Work out the finished part from the listing and answer in its coordinate system (mm). Face numbers are marked on the shaded views. A direction names the side the tool comes from. Coordinates: 2 decimals unless noted, no trailing zeros. Write each loop counter-clockwise with the first axis right and the second up, starting at its lowest first coordinate (ties: lowest second). Pieces come first, ordered by that corner, then holes. Notation, with made-up numbers: (35.5, -8) - (78.5, -8) arc R14 ccw to (78.5, 11) - close; hole circle Ø8 at (0, 39.25). An arc over 180 degrees is marked (long way). One line per item, written item: value.
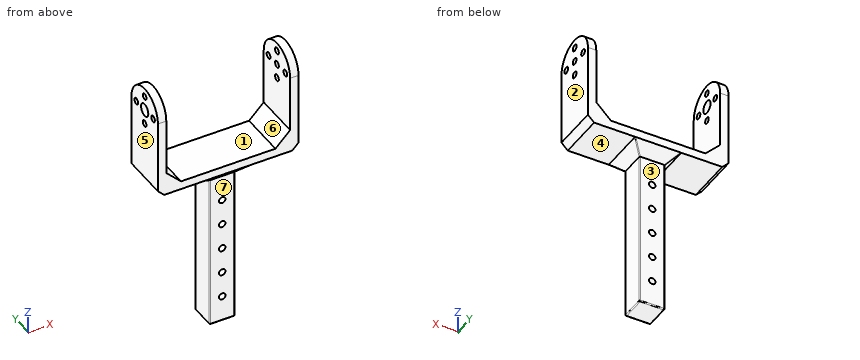
```python
from build123d import *

# Parameters (mm, degrees)
BOSS_EXTRUDE1_DEPTH      = 22
SKETCH3_R                = 1.55
CUT_EXTRUDE1_DEPTH       = 30
CUT_EXTRUDE5_DEPTH       = 9
SKETCH11_R               = 1.55
CUT_EXTRUDE10_DEPTH      = 13
CUT_EXTRUDE11_START      = -10
CUT_EXTRUDE11_DEPTH      = 10
SKETCH13_R               = 3
SKETCH13_R_2             = 1.5
CUT_EXTRUDE12_DEPTH      = 4
SKETCH14_W               = 54
SKETCH14_H               = 9.3
SKETCH14_W_2             = 7.05
SKETCH14_H_2             = 4
BOSS_EXTRUDE4_DEPTH      = 4
SKETCH17_W               = 7.05
SKETCH17_H               = 4
BOSS_EXTRUDE5_DEPTH      = 23.05
BOSS_EXTRUDE6_DEPTH      = 27.3
BOSS_EXTRUDE6_DEPTH_BACK = 4
SKETCH18_W               = 54
SKETCH18_H               = 2.95
SKETCH19_W               = 54
SKETCH19_H               = 2.8
BOSS_EXTRUDE7_DEPTH      = 21
FILLET2_SIZE             = 6.5
FILLET3_SIZE             = 0.5
SKETCH20_R               = 3.970030919
BOSS_EXTRUDE8_DEPTH      = 6
FILLET4_R                = 1
CUT_EXTRUDE13_START      = -37.3
CUT_EXTRUDE13_DEPTH      = 37.3
SKETCH22_W               = 56.118071471
SKETCH22_H               = 11.813110758
CUT_EXTRUDE14_DEPTH      = 56
SKETCH23_W               = 67
SKETCH23_H               = 4
BOSS_EXTRUDE9_DEPTH      = 4
SKETCH24_W               = 67
SKETCH24_H               = 4
BOSS_EXTRUDE10_DEPTH     = 4
SKETCH25_W               = 12
SKETCH25_H               = 12
BOSS_EXTRUDE11_DEPTH     = 80
FILLET6_SIZE             = 7
SKETCH27_W               = 67
SKETCH27_H               = 4
CUT_EXTRUDE16_DEPTH      = 80
FILLET7_SIZE             = 5
SKETCH29_R               = 1.55
CUT_EXTRUDE17_DEPTH      = 12
FILLET8_R                = 0.5
FILLET9_R                = 0.5
FILLET10_SIZE            = 3


# Read off the part's stored shape, not the designer's step: Cut-Extrude13
with BuildPart() as part:
    # Sketch1 → Boss-Extrude1 (new body)
    with BuildSketch(Plane(origin=(0, 0, 0), x_dir=(1, 0, 0), z_dir=(0, 1, 0))):
        Polygon((0, 0), (0, 50), (67, 50), (67, 0), (63, 0), (63, 46), (4, 46), (4, 0), align=None)
    extrude(amount=BOSS_EXTRUDE1_DEPTH)

    # Sketch3 → Cut-Extrude1 (cut)
    with BuildSketch(Plane(origin=(67, 0, 0), x_dir=(0, 0, -1), z_dir=(1, 0, 0))):
        with Locations((12.05, 11)):
            Circle(SKETCH3_R)
    extrude(amount=-CUT_EXTRUDE1_DEPTH, mode=Mode.SUBTRACT)

    # Sketch5 → Cut-Extrude5 (cut)
    with BuildSketch(Plane(origin=(67, 0, 0), x_dir=(0, 0, -1), z_dir=(1, 0, 0))):
        with BuildLine():
            Line((12.05, 22), (0, 22))
            Line((0, 22), (0, 0))
            Line((0, 0), (12.05, 0))
            ThreePointArc((12.05, 0), (1.05, 11), (12.05, 22))
        make_face()
    extrude(amount=-CUT_EXTRUDE5_DEPTH, mode=Mode.SUBTRACT)

    # Sketch11 → Cut-Extrude10 (cut)
    with BuildSketch(Plane(origin=(67, 0, 0), x_dir=(0, 0, -1), z_dir=(1, 0, 0))):
        with Locations((19.05, 11)):
            Circle(SKETCH11_R)
        with Locations((12.05, 18)):
            Circle(SKETCH11_R)
        with Locations((12.05, 4)):
            Circle(SKETCH11_R)
        with Locations((5.05, 11)):
            Circle(SKETCH11_R)
    extrude(amount=-CUT_EXTRUDE10_DEPTH, mode=Mode.SUBTRACT)

    # Sketch12 → Cut-Extrude11 (cut)
    with BuildSketch(Plane.ZY.offset(CUT_EXTRUDE11_START)):
        with BuildLine():
            Line((-12.05, 22), (0, 22))
            Line((0, 22), (0, 0))
            Line((0, 0), (-12.05, 0))
            ThreePointArc((-12.05, 0), (-1.05, 11), (-12.05, 22))
        make_face()
    extrude(amount=CUT_EXTRUDE11_DEPTH, mode=Mode.SUBTRACT)

    # Sketch13 → Cut-Extrude12 (cut)
    with BuildSketch(Plane.ZY):
        with Locations((-12.05, 11)):
            Circle(SKETCH13_R)
        with Locations((-19.05, 11)):
            Circle(SKETCH13_R_2)
        with Locations((-12.05, 4)):
            Circle(SKETCH13_R_2)
        with Locations((-5.05, 11)):
            Circle(SKETCH13_R_2)
        with Locations((-12.05, 18)):
            Circle(SKETCH13_R_2)
    extrude(amount=-CUT_EXTRUDE12_DEPTH, mode=Mode.SUBTRACT)

    # Sketch14 → Boss-Extrude4 (add)
    with BuildSketch(Plane(origin=(0, 0, -50), x_dir=(-1, 0, 0), z_dir=(0, 0, -1))):
        with Locations((-33.5, -4.65)):
            Rectangle(SKETCH14_W, SKETCH14_H)
        with Locations((-56.975, 20)):
            Rectangle(SKETCH14_W_2, SKETCH14_H_2)
        with Locations((-10.025, 20)):
            Rectangle(SKETCH14_W_2, SKETCH14_H_2)
    extrude(amount=-BOSS_EXTRUDE4_DEPTH)

    # Sketch17 → Boss-Extrude5 (add)
    with BuildSketch(Plane(origin=(0, 0, -50), x_dir=(-1, 0, 0), z_dir=(0, 0, -1))):
        with Locations((-56.975, 20)):
            Rectangle(SKETCH17_W, SKETCH17_H)
        with Locations((-10.025, 20)):
            Rectangle(SKETCH17_W, SKETCH17_H)
    extrude(amount=BOSS_EXTRUDE5_DEPTH)

    # Sketch18 → Boss-Extrude6 (add, two sides: drawn at the far end of the back side and taken through both)
    with BuildSketch(Plane.XZ.offset(-18).offset(-BOSS_EXTRUDE6_DEPTH_BACK)):
        with Locations((33.5, -71.575)):
            Rectangle(SKETCH18_W, SKETCH18_H)
    extrude(amount=BOSS_EXTRUDE6_DEPTH + BOSS_EXTRUDE6_DEPTH_BACK)

    # Sketch19 → Boss-Extrude7 (add)
    with BuildSketch(Plane(origin=(0, 0, -50), x_dir=(-1, 0, 0), z_dir=(0, 0, -1))):
        with Locations((-33.5, -7.9)):
            Rectangle(SKETCH19_W, SKETCH19_H)
    extrude(amount=BOSS_EXTRUDE7_DEPTH)

    # Fillet2
    fillet2_edges = [part.edges().sort_by_distance(p)[0] for p in [
        (60.5, 20, -50),
        (6.5, 20, -50),
    ]]
    chamfer(fillet2_edges, length=FILLET2_SIZE - 0.0001)  # a hair under: the kernel refuses the full size

    # Fillet3
    fillet3_edges = [part.edges().sort_by_distance(p)[0] for p in [
        (60.5, 6.35, -73.05),
        (6.5, 6.35, -73.05),
    ]]
    chamfer(fillet3_edges, length=FILLET3_SIZE)

    # Sketch20 → Boss-Extrude8 (add)
    with BuildSketch(Plane.XZ.offset(9.3)):
        with Locations(Location((23.4, -59.65, 0), (0, 0, 270))):
            Circle(SKETCH20_R)
    extrude(amount=BOSS_EXTRUDE8_DEPTH)

    # Fillet4
    fillet4_edges = [part.edges().sort_by_distance(p)[0] for p in [
        (23.4, -15.3, -55.679969081),
    ]]
    fillet(fillet4_edges, radius=FILLET4_R)

    # Cut-Extrude13 outline → Cut-Extrude13 (cut)
    with BuildSketch(Plane(origin=(0, 22, 0), x_dir=(1, 0, 0), z_dir=(0, 1, 0)).offset(CUT_EXTRUDE13_START)):
        Polygon((67, 50), (60.5, 56.5), (60.5, 72.55), (60, 73.05), (7, 73.05), (6.5, 72.55), (6.5, 56.5), (0, 50), align=None)
    extrude(amount=CUT_EXTRUDE13_DEPTH, mode=Mode.SUBTRACT)

    # Sketch22 → Cut-Extrude14 (cut)
    with BuildSketch(Plane(origin=(0, 0, -50), x_dir=(-1, 0, 0), z_dir=(0, 0, -1))):
        with Locations((-32.440964265, -5.906555379)):
            Rectangle(SKETCH22_W, SKETCH22_H)
    extrude(amount=-CUT_EXTRUDE14_DEPTH, mode=Mode.SUBTRACT)

    # Sketch23 → Boss-Extrude9 (add)
    with BuildSketch(Plane(origin=(0, 22, 0), x_dir=(1, 0, 0), z_dir=(0, 1, 0))):
        with Locations((33.5, 48)):
            Rectangle(SKETCH23_W, SKETCH23_H)
    extrude(amount=BOSS_EXTRUDE9_DEPTH)

    # Sketch24 → Boss-Extrude10 (add)
    with BuildSketch(Plane.XZ):
        with Locations((33.5, -48)):
            Rectangle(SKETCH24_W, SKETCH24_H)
    extrude(amount=BOSS_EXTRUDE10_DEPTH)

    # Sketch25 → Boss-Extrude11 (add)
    with BuildSketch(Plane(origin=(0, 0, -50), x_dir=(-1, 0, 0), z_dir=(0, 0, -1))):
        with Locations((-33.5, 11)):
            Rectangle(SKETCH25_W, SKETCH25_H)
    extrude(amount=BOSS_EXTRUDE11_DEPTH)

    # Fillet6
    fillet6_edges = [part.edges().sort_by_distance(p)[0] for p in [
        (63, 11, -46),
        (4, 11, -46),
    ]]
    chamfer(fillet6_edges, length=FILLET6_SIZE)

    # Sketch27 → Cut-Extrude16 (cut)
    with BuildSketch(Plane.XY.offset(-46)):
        with Locations((33.5, 24)):
            Rectangle(SKETCH27_W, SKETCH27_H)
        with Locations((33.5, -2)):
            Rectangle(SKETCH27_W, SKETCH27_H)
    extrude(amount=-CUT_EXTRUDE16_DEPTH, mode=Mode.SUBTRACT)

    # Fillet7
    fillet7_edges = [part.edges().sort_by_distance(p)[0] for p in [
        (39.5, 11, -50),
        (33.5, 5, -50),
        (27.5, 11, -50),
        (33.5, 17, -50),
    ]]
    chamfer(fillet7_edges, length=FILLET7_SIZE - 0.0001)  # a hair under: the kernel refuses the full size

    # Sketch29 → Cut-Extrude17 (cut)
    with BuildSketch(Plane.XZ.offset(-5)):
        with Locations(Location((33.5, -67.5, 0), (0, 0, 270))):
            Circle(SKETCH29_R)
        with Locations(Location((33.5, -80, 0), (0, 0, 270))):
            Circle(SKETCH29_R)
        with Locations(Location((33.5, -92.5, 0), (0, 0, 270))):
            Circle(SKETCH29_R)
        with Locations(Location((33.5, -105, 0), (0, 0, 270))):
            Circle(SKETCH29_R)
        with Locations(Location((33.5, -117.5, 0), (0, 0, 270))):
            Circle(SKETCH29_R)
    extrude(amount=-CUT_EXTRUDE17_DEPTH, mode=Mode.SUBTRACT)

    # Fillet8
    fillet8_edges = [part.edges().sort_by_distance(p)[0] for p in [
        (39.5, 17, -92.49995),
        (39.5, 5, -92.49995),
        (27.5, 5, -92.49995),
        (27.5, 17, -92.49995),
        (39.5, 11, -130),
        (33.5, 5, -130),
        (27.5, 11, -130),
        (33.5, 17, -130),
    ]]
    fillet(fillet8_edges, radius=FILLET8_R)

    # Fillet9
    fillet9_edges = [part.edges().sort_by_distance(p)[0] for p in [
        (41.926726695, 19.426726695, -52.573173305),
        (41.926726695, 2.573273305, -52.573173305),
        (25.073273305, 19.426726695, -52.573173305),
        (25.073273305, 2.573273305, -52.573173305),
    ]]
    fillet(fillet9_edges, radius=FILLET9_R)

    # Fillet10
    fillet10_edges = [part.edges().sort_by_distance(p)[0] for p in [
        (0, 11, -50),
        (67, 11, -50),
    ]]
    chamfer(fillet10_edges, length=FILLET10_SIZE)


solid = part.part
```
Item 1: Section A-A, the plane z = -28 is taken. Determine the outline of the cut face in (x, y), then the cut area to 3 significant figures.
Evaluation:
outline: (0, 0) - (4, 0) - (4, 22) - (0, 22) - close; (63, 0) - (67, 0) - (67, 22) - (63, 22) - close
area: 176 mm2
Item 2: Section B-B, the plane z = -101 is taken. Determine the outline of the cut face in (x, y), then the cut area to 3 significant figures.
Evaluation:
outline: (27.5, 5.5) arc R0.5 ccw to (28, 5) - (39, 5) arc R0.5 ccw to (39.5, 5.5) - (39.5, 16.5) arc R0.5 ccw to (39, 17) - (28, 17) arc R0.5 ccw to (27.5, 16.5) - close
area: 144 mm2
Item 3: Section D-D, the plane z = -117.5 is taken. Determine the outline of the cut face in (x, y).
Evaluation:
outline: (27.5, 5.5) arc R0.5 ccw to (28, 5) - (31.95, 5) - (31.95, 17) - (28, 17) arc R0.5 ccw to (27.5, 16.5) - close; (35.05, 5) - (39, 5) arc R0.5 ccw to (39.5, 5.5) - (39.5, 16.5) arc R0.5 ccw to (39, 17) - (35.05, 17) - close
Item 4: Section C-C, the plane z = -44 is taken. Determine the outline of the cut face in (x, y), then the cut area to 3 significant figures.
Evaluation:
outline: (0, 0) - (9, 0) - (9, 22) - (0, 22) - close; (58, 0) - (67, 0) - (67, 22) - (58, 22) - close
area: 396 mm2
Item 5: Which of the six approach directions +Z, -Z, +X, -X, +Y, -Y give full straight-line access (tool end or side, diameter ignored) to the marked faces 4, 5, 6 and 7?
Evaluation:
face 4: -Z, +Y, -Y
face 5: +Z, -Z, -X, +Y, -Y
face 6: +Z, +Y, -Y
face 7: -Z, +X, -X, -Y
Item 6: Determine the mould class of the marked faces 1, 2 and 3 for opening direction X: +X half, -X half, draft (parallel to the pull), parting line (faces both ways), or undercut.
Evaluation:
face 1: undercut
face 2: +X half
face 3: draft
Item 7: Given pin 1 (1.5 mm diameter, centred on x = 20, y = 14.5, fed in from +Z); pin 2 (1.9 mm diameter, centred on y = 4, z = -12.05, fed in from -X); pin 3 (10 mm diameter, centred on x = 59, y = 9, fed in from -Z); pin 4 (4 mm diameter, centred on y = 17, z = -69, fed in from -X), each flat-ended and moving along its own axis, determine where each tip first touches the part or whether it passes through.
Evaluation:
pin 1: stops at z = -46
pin 2: passes through
pin 3: stops at z = -50
pin 4: stops at x = 27.5
Item 8: Consider probe 1 along Y at (x, z) = (64.9, -12.05); probe 2 along Y at (x, z) = (2.3, -12.05); probe 3 along X at (y, z) = (20, -8.5). Determine where each line is inside the solid, lowest interval first.
Evaluation:
probe 1: y = 0 to 2.45, 5.55 to 9.45, 12.55 to 16.45, 19.55 to 22
probe 2: y = 0 to 2.5, 5.5 to 8, 14 to 16.5, 19.5 to 22
probe 3: x = 0 to 4, 63 to 67
